For this review, use the dimensioned drawing (mm, ordinates from the lowest corner) and the shaded views. A direction names the side the tool comes from. Coordinates: 2 decimals unless noted, no trailing zeros. Loops run counter-clockwise (first coordinate to the right, second up) from the corner with the lowest first, then second, coordinate; pieces in that order, holes last. Notation, with made-up numbers: (72.25, 16.25) - (102.25, 16.25) arc R19 cw to (102.25, 50.25) - close; hole circle Ø4 at (64.5, -21). An arc over 180 degrees is marked (long way). Answer in a Markdown table with one row per item. Add a question column.
(1) We need section A-A, the plane z = 8. Write out the cut boundary in (x, y) (1 decimal).
(2) We need section C-C, the plane z = 10.25. Write out the cut boundary in (x, y) (1 decimal), plus the area to 3 significant figures.
(3) The part is to be moulded in two halves that separate along X. For the marked faces 5, 6 and 7, say which applies: released by +X, released by -X, zero draft, split by the parting line, or undercut.
(4) For the marked faces 1, 2, 3 and 4, list the 3-axis set-ups (+Z, -Z, +X, -X, +Y, -Y) from which the entire face can be reached by the end or side of a thin tool; tool diameter is ignored.
(5) We need section B-B, the plane x = 10. Write out the cut boundary in (y, z).
(6) Clearance check with flat-ended pins moving along their axes: pin 1 (3.5 mm diameter, centred on x = 10, z = 8, fed in from -Y); pin 2 (1.2 mm diameter, centred on x = 5.5, y = 10, fed in from +Z); pin 3 (2 mm diameter, centred on y = 14, z = 5, fed in from +X). State where each tip first meets the part, or that it passes through.
(7) To check wall thickness, follow L1, parallel to Z at x = 10, y = 5.9; L2, parallel to Y at x = 12, z = 6.75; L3, parallel to Z at x = 12.5, y = 3.75. State the ranges of each line that lie inside material, in increasing order. Write a range as [from, to].
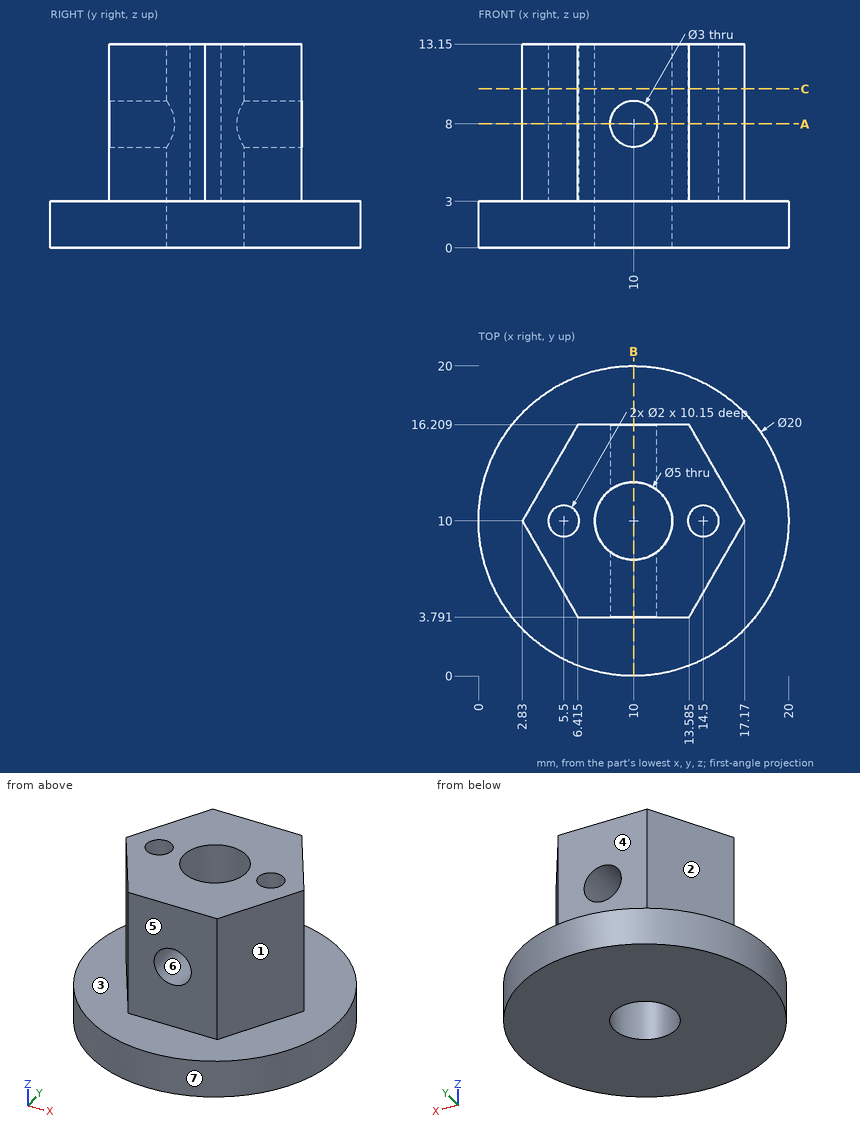
Responses:
| question | item | result |
|---|---|---|
| 1 | outline | (2.8, 10) - (6.4, 3.8) - (8.5, 3.8) - (8.5, 8) arc R2.5 cw to (8.5, 12) - (8.5, 16.2) - (6.4, 16.2) - close; (11.5, 3.8) - (13.6, 3.8) - (17.2, 10) - (13.6, 16.2) - (11.5, 16.2) - (11.5, 12) arc R2.5 cw to (11.5, 8) - close; hole circle Ø2 at (5.5, 10); hole circle Ø2 at (14.5, 10) |
| 2 | outline | (2.8, 10) - (6.4, 3.8) - (13.6, 3.8) - (17.2, 10) - (13.6, 16.2) - (6.4, 16.2) - close; hole circle Ø2 at (5.5, 10); hole circle Ø5 at (10, 10); hole circle Ø2 at (14.5, 10) |
| 2 | area | 108 mm2 |
| 3 | face 5 | zero draft |
| 3 | face 6 | undercut |
| 3 | face 7 | split by the parting line |
| 4 | face 1 | +Z, +X, -Y |
| 4 | face 2 | +Z, -X, +Y |
| 4 | face 3 | +Z |
| 4 | face 4 | +Z, +X, -X, +Y |
| 5 | outline | (0, 0) - (7.5, 0) - (7.5, 6.5) - (3.79, 6.5) - (3.79, 3) - (0, 3) - close; (3.79, 9.5) - (7.5, 9.5) - (7.5, 13.15) - (3.79, 13.15) - close; (12.5, 0) - (20, 0) - (20, 3) - (16.21, 3) - (16.21, 6.5) - (12.5, 6.5) - close; (12.5, 9.5) - (16.21, 9.5) - (16.21, 13.15) - (12.5, 13.15) - close |
| 6 | pin 1 | stops at y = 3.79 |
| 6 | pin 2 | stops at z = 3 |
| 6 | pin 3 | stops at x = 15.44 |
| 7 | L1 | z = [0, 6.5], [9.5, 13.15] |
| 7 | L2 | y = [3.79, 8.5], [11.5, 16.21] |
| 7 | L3 | z = [0, 3] |
